Autodesk Inventor part; units mm, degrees
ref_plane "XZ Plane" through (0, 0, 0) normal (0, 1, 0) x (-1, 0, 0)
ref_plane "XY Plane" through (0, 0, 0) normal (0, 0, 1) x (1, 0, 0)
sketch "Sketch1" plane through (0, 0, 0) normal (0, 0, 1) x (1, 0, 0)
  line L0 (29.845, -31.115) -> (-29.845, -31.115)
  line L1 (-29.845, -31.115) -> (-29.845, 31.115)
  line L2 (-29.845, 31.115) -> (29.845, 31.115)
  line L3 (29.845, 31.115) -> (29.845, -31.115)
  line L4 (29.845, -31.115) -> (-29.845, 31.115) construction
  line L5 (-29.845, -31.115) -> (29.845, 31.115) construction
  point P0 (0, 0)
  dimension "d0" = 59.69
  dimension "d1" = 62.23
extrude "Extrusion1" add sketch "Sketch1" along normal blind 28.575
sketch "Sketch2" plane through (-29.845, 31.115, 0) normal (0, 1, 0) x (1, 0, 0)
  line L0 (0, 0) -> (59.69, 0)
  line L1 (59.69, 0) -> (59.69, -28.575)
  line L2 (56.134, 0) -> (25.88, 0)
  line L3 (25.88, 0) -> (25.88, -3.175)
  line L4 (25.88, -3.175) -> (56.134, -3.175)
  line L5 (59.69, 0) -> (0, 0)
  line L6 (56.134, 0) -> (56.134, -3.175)
  point P0 (29.845, 0)
  dimension "d4" = 3.175
  dimension "d5" = 30.254
  dimension "d52" = 3.556
extrude "Extrusion2" cut sketch "Sketch2" against normal blind 38.735
sketch "Sketch3" plane through (0, 0, 0) normal (0, 0, 1) x (1, 0, 0)
  point P0 (0, 0)
sketch "Sketch4" plane through (0, 0, 28.575) normal (0, 0, 1) x (1, 0, 0)
  line L0 (0.535, 7.4422) -> (21.535, 7.4422) construction
  line L1 (21.535, 7.4422) -> (21.535, 19.4422) construction
  line L2 (21.535, 19.4422) -> (0.535, 19.4422) construction
  line L3 (0.535, 19.4422) -> (0.535, 7.4422) construction
  line L4 (-29.845, -31.115) -> (29.845, -31.115)
  line L5 (-3.965, 31.115) -> (-3.965, -7.62)
  point P0 (0, 0)
  dimension "d8" = 21
  dimension "d9" = 12
  dimension "d10" = 38.5572
  dimension "d11" = 4.5
hole "Hole1" at (0.535, 19.4422, 28.575) at (0.535, 7.4422, 28.575) at (21.535, 7.4422, 28.575) at (21.535, 19.4422, 28.575) direction (0, 0, -1) diameter 2.8702 end through all counterbore diameter 6.35 counterbore depth 21.209
fillet "Fillet1" radius 3.175 2 edges at (-3.965, -7.62, 1.5875) (26.289, -7.62, 1.5875)
sketch "Sketch5" plane through (29.845, -31.115, 28.575) normal (1, 0, 0) x (0, 0, -1)
  line L0 (0, 0) -> (12.7, 0)
  line L1 (12.7, 0) -> (12.7, 10.16)
  line L2 (12.7, 10.16) -> (0, 10.16)
  line L3 (0, 10.16) -> (0, 0)
  point P0 (28.575, 31.115)
  dimension "d20" = 12.7
  dimension "d21" = 10.16
extrude "Extrusion3" add sketch "Sketch5" along normal blind 12.7
sketch "Sketch6" plane through (-29.845, -31.115, 0) normal (0, -1, 0) x (1, 0, 0)
  line L0 (29.845, 34.29) -> (29.845, -5.715)
  line L1 (0, 28.575) -> (72.39, 28.575)
  line L2 (72.39, 28.575) -> (72.39, 15.875)
  line L3 (0, 0) -> (0, 28.575)
  point P0 (67.0052, 22.225)
  point P1 (5.4102, 22.225)
  point P2 (5.4102, 5.715)
  dimension "d39" = 6.35
  dimension "d40" = 37.1602
  dimension "d41" = 16.51
  dimension "d42" = 61.595
  dimension "d67" = 5.3848
  dimension "d68" = 5.4102
hole "Hole2" at (37.1602, -31.115, 22.225) at (-24.4348, -31.115, 22.225) at (-24.4348, -31.115, 5.715) direction (0, 1, 0) diameter 5.7912 depth 12.7 tip angle 118
sketch "Sketch7" plane through (0, 0, 0) normal (0, 0, 1) x (1, 0, 0)
  line L0 (29.845, -20.955) -> (42.545, -20.955)
  line L1 (-29.845, 31.115) -> (-29.845, -31.115)
  line L2 (-29.845, -31.115) -> (42.545, -31.115)
  line L3 (29.845, 31.115) -> (-29.845, 31.115)
  line L4 (-29.845, -20.955) -> (-19.2024, -20.955)
  line L5 (-19.2024, -20.955) -> (-19.2024, 31.115)
  line L6 (-19.2024, 31.115) -> (-29.845, 31.115)
  line L7 (-29.845, 31.115) -> (-29.845, -20.955)
  point P0 (0, 0)
  dimension "d35" = 10.6426
  dimension "d36" = 10.16
  dimension "d43" = 0
extrude "Extrusion4" cut sketch "Sketch7" along normal up to next
sketch "Sketch8" plane through (-29.845, -20.955, 28.575) normal (0, 1, 0) x (1, 0, 0)
  circle A0 centre (5.4102, 22.86) radius 2.8956
  point P0 (29.845, 28.575)
sketch "Sketch9" plane through (-29.845, -31.115, 0) normal (0, -1, 0) x (1, 0, 0)
  line L0 (59.69, 15.875) -> (72.39, 15.875)
  line L1 (59.69, 0) -> (59.69, 15.875)
  line L2 (59.69, 0) -> (59.69, 28.575) construction
  line L3 (59.69, 15.875) -> (45.72, 15.875)
  line L4 (45.72, 15.875) -> (45.72, 3.175)
  line L5 (45.72, 3.175) -> (59.69, 3.175)
  line L6 (59.69, 3.175) -> (59.69, 15.875)
  line L7 (59.69, 0) -> (0, 0) construction
  point P0 (29.845, 0)
  point P1 (59.69, 3.175)
  dimension "d44" = 13.97
  dimension "d46" = 0
  dimension "d48" = 3.175
extrude "Extrusion5" cut sketch "Sketch9" against normal blind 15.24
fillet "Fillet2" radius 3.175 2 edges at (15.875, -23.495, 3.175) (15.875, -23.495, 15.875)
sketch "Sketch10" plane through (0, 0, 0) normal (0, 0, -1) x (-1, 0, 0)
  line L0 (-29.845, 31.115) -> (-29.845, -31.115)
  line L1 (-26.289, 31.115) -> (-29.845, 31.115)
  line L2 (-26.289, -4.445) -> (-26.289, 31.115)
  line L3 (-29.845, 31.115) -> (-26.289, 31.115)
  line L4 (-26.289, 31.115) -> (-26.289, -2.54)
  line L5 (-26.289, -2.54) -> (-29.845, -2.54)
  line L6 (-29.845, -2.54) -> (-29.845, 31.115)
  point P0 (0, 0)
  dimension "d53" = 33.655
extrude "Extrusion6" add sketch "Sketch10" along normal blind 2.54
sketch "Sketch11" plane through (29.845, -20.955, 28.575) normal (1, 0, 0) x (0, 0, -1)
  line L0 (0, 52.07) -> (31.115, 52.07)
  line L1 (31.115, 52.07) -> (31.115, 18.415)
  point P0 (28.575, 20.955)
  point P1 (27.94, 46.6852)
  point P2 (27.94, 22.098)
  point P3 (27.94, 34.3916)
  dimension "d56" = 3.175
  dimension "d57" = 5.3848
  dimension "d58" = 24.5872
  dimension "d66" = 12.2936
hole "Hole3" at (29.845, 25.7302, 0.635) at (29.845, 1.143, 0.635) at (29.845, 13.4366, 0.635) direction (-1, 0, 0) diameter 2.4638 end up to surface
properties part number "J005333" material "ALUMINUM, 6061-T651"
For this review, take the finished solid that the model builds, in its own axes (mm). A direction names the side the tool comes from. Coordinates: 2 decimals unless noted, no trailing zeros. Loops run counter-clockwise (first coordinate to the right, second up) from the corner with the lowest first, then second, coordinate; pieces in that order, holes last. Notation, with made-up numbers: (47.5, 66.25) - (65.5, 66.25) arc R36 ccw to (65.5, 100.25) - close; hole circle Ø2 at (19.25, 36). An arc over 180 degrees is marked (long way). Use one line per item in the form item = value. Start each with the question number.
1) To check wall thickness, follow probe 1 along X at (y, z) = (20.5, 4) (3 decimals); probe 2 along Y at (x, z) = (19.5, 14) (3 decimals); probe 3 along X at (y, z) = (6, 17) (3 decimals). State the ranges of each line that lie inside material, in increasing order. Write a range as from..to.
2) For pin 1 (6.5 mm diameter, centred on y = 21.5, z = -1, fed in from -X); pin 2 (2.5 mm diameter, centred on x = 14.5, z = 1, fed in from +Y); pin 3 (4 mm diameter, centred on y = -18.5, z = 17.5, fed in from +X) (3 decimals), all flat-tipped, find the tip position at first contact; note any pin that passes through.
3) For faces 4 (the face through (16.83, -23.39, 4.08)), 5 (the face through (-1, 7, 7.366)), 6 (the face through (11, 12, 3.175)), list the 3-axis set-ups (+Z, -Z, +X, -X, +Y, -Y) from which the entire face can be reached by the end or side of a thin tool; tool diameter is ignored.
4) Draft analysis for pull direction Y (two halves, no side actions). For faces 1 (the face through (39.987, -25.964, 22.853)), 2 (the face through (20.565, 8.5, 5.241)), 3 (the face through (5, 31.115, 17)), state which applies: released by +Y, released by -Y, zero draft, split by the parting line, or undercut.
5) Take a section at D-D (x = -23.5). State the section outline as (y, z) points (3 decimals), plus the area to 3 significant figures.
6) Take a section at C-C (y = 20). State the section outline as (x, z) points (3 decimals).
7) Take a section at A-A (z = 4). State the section outline as (x, y) points (3 decimals), plus the area to 3 significant figures.
8) Take a section at B-B (z = 18). State the section outline as (x, y) points (3 decimals).
From the geometry:
q1.probe_1 = -19.202..-0.435, 1.505..20.565, 22.505..29.845
q1.probe_2 = -15.875..5.005, 9.879..17.005, 21.879..31.115
q1.probe_3 = -19.202..-2.294, 3.364..18.706, 24.364..29.845
q2.pin_1 = -19.2
q2.pin_2 = -7.62
q2.pin_3 = 29.845
q3.face_4 = +X, -Y
q3.face_5 = +Z
q3.face_6 = -Z, +Y
q4.face_1 = zero draft
q4.face_2 = undercut
q4.face_3 = released by +Y
q5.outline = (-31.115, 0) - (-20.955, 0) - (-20.955, 2.974) - (-31.115, 2.974) - close; (-31.115, 8.456) - (-20.955, 8.456) - (-20.955, 19.484) - (-31.115, 19.484) - close; (-31.115, 24.966) - (-20.955, 24.966) - (-20.955, 28.575) - (-31.115, 28.575) - close
q5.area = 179 mm2
q6.outline = (-19.202, 0) - (-3.965, 0) - (-3.965, 3.175) - (-0.787, 3.175) - (-0.787, 7.366) - (-2.591, 7.366) - (-2.591, 28.575) - (-19.202, 28.575) - close; (1.857, 3.175) - (20.213, 3.175) - (20.213, 7.366) - (18.409, 7.366) - (18.409, 28.575) - (3.661, 28.575) - (3.661, 7.366) - (1.857, 7.366) - close; (22.857, 3.175) - (26.289, 3.175) - (26.289, -2.54) - (29.845, -2.54) - (29.845, 28.575) - (24.661, 28.575) - (24.661, 7.366) - (22.857, 7.366) - close
q7.outline = (-29.845, -31.115) - (-26.768, -31.115) - (-26.768, -20.955) - (-29.845, -20.955) - close; (-22.102, -31.115) - (16.915, -31.115) - (16.915, -15.875) - (29.845, -15.875) - (29.845, 31.115) - (-19.202, 31.115) - (-19.202, -20.955) - (-22.102, -20.955) - close; hole circle Ø2.87 at (0.535, 7.442); hole circle Ø2.87 at (0.535, 19.442); hole circle Ø2.87 at (21.535, 7.442); hole circle Ø2.87 at (21.535, 19.442)
q7.area = 2,890 mm2
q8.outline = (-29.845, -31.115) - (42.545, -31.115) - (42.545, -20.955) - (29.845, -20.955) - (29.845, 31.115) - (-19.202, 31.115) - (-19.202, -20.955) - (-29.845, -20.955) - close; hole circle Ø6.35 at (0.535, 7.442); hole circle Ø6.35 at (0.535, 19.442); hole circle Ø6.35 at (21.535, 7.442); hole circle Ø6.35 at (21.535, 19.442)
